```python
from build123d import *

# Parameters (mm, degrees)
SKETCH1_R           = 7.239
SKETCH1_W           = 3.175
SKETCH1_H           = 3.175
BOSS_EXTRUDE1_DEPTH = 6.35
SKETCH2_R           = 7.239
SKETCH2_W           = 3.175
SKETCH2_H           = 3.175
BOSS_EXTRUDE2_DEPTH = 0.254
SKETCH3_R           = 7.239
BOSS_EXTRUDE3_DEPTH = 6.35


with BuildPart() as part:
    # Sketch1 → Boss-Extrude1 (new body)
    with BuildSketch(Plane(origin=(0, 0, 0), x_dir=(1, 0, 0), z_dir=(0, 1, 0))):
        Circle(SKETCH1_R)
        Rectangle(SKETCH1_W, SKETCH1_H, mode=Mode.SUBTRACT)
    extrude(amount=BOSS_EXTRUDE1_DEPTH)

    # Sketch2 → Boss-Extrude2 (add)
    with BuildSketch(Plane(origin=(0, 6.35, 0), x_dir=(1, 0, 0), z_dir=(0, 1, 0))):
        Circle(SKETCH2_R)
        Rectangle(SKETCH2_W, SKETCH2_H, mode=Mode.SUBTRACT)
        Rectangle(SKETCH2_W, SKETCH2_H)
    extrude(amount=BOSS_EXTRUDE2_DEPTH)

    # Sketch3 → Boss-Extrude3 (add)
    with BuildSketch(Plane(origin=(0, 6.604, 0), x_dir=(1, 0, 0), z_dir=(0, 1, 0))):
        Circle(SKETCH3_R)
        Polygon((-1, -1), (-3, -1), (-3, 1), (-1, 1), (-1, 3), (1, 3), (1, 1), (3, 1), (3, -1), (1, -1), (1, -3), (-1, -3), align=None, mode=Mode.SUBTRACT)
    extrude(amount=BOSS_EXTRUDE3_DEPTH)


solid = part.part
```
Work out the finished part from the listing and answer in its coordinate system (mm). A direction names the side the tool comes from. Coordinates: 2 decimals unless noted, no trailing zeros. Order: outer loops, then holes, each group sorted by start corner. A loop starts at its lowest first (then second) coordinate and runs counter-clockwise, first axis right, second up. Notation, with made-up numbers: M -32,-35.5 L 10,-35.5 A28 cw 10,-11.5 Z; hole C -11,-26.5 d2. An arc over 180 degrees is marked long. Use CSV: the item, a comma, the result in double quotes.
1) For faces 4 (the face through (1.588, 3, 0)), 5 (the face through (-2, 0, 0)), 6 (the face through (-2, 10, -1)), determine the directions among +Z, -Z, +X, -X, +Y, -Y from which every point of the face is accessible in a straight line to the end or side of a thin tool.
Worked out:
face 4,"-Y"
face 5,"+Z, -Z, +X, -X, -Y"
face 6,"+Y"
2) Consider line 1 (X direction, y = 10, z = 0.25); line 2 (X direction, y = 7, z = 1.75); line 3 (Y direction, x = 2.75, z = -0.5). Determine where each line is inside the solid, lowest interval first. Write a range as [from, to].
Worked out:
line 1,"x = [-7.23, -3], [3, 7.23]"
line 2,"x = [-7.02, -1], [1, 7.02]"
line 3,"y = [0, 6.6]"
3) Determine the mould class of faces 1 (the face through (-3, 10, 0)), 2 (the face through (2, 12.954, 2)), 3 (the face through (-0.942, 6.386, -7.177)) for opening direction Z: released by +Z, released by -Z, zero draft, split by the parting line, or undercut.
Worked out:
face 1,"undercut"
face 2,"zero draft"
face 3,"split by the parting line"
4) Section B-B on y = 12.25 is taken. Write down the section's boundary in (x, z).
Worked out:
outline,"C 0,0 d14.48; hole M -3,-1 L -1,-1 L -1,-3 L 1,-3 L 1,-1 L 3,-1 L 3,1 L 1,1 L 1,3 L -1,3 L -1,1 L -3,1 Z"
5) Section A-A on z = 0 is taken. Write down the section's boundary in (x, y).
Worked out:
outline,"M -7.24,0 L -1.59,0 L -1.59,6.35 L 1.59,6.35 L 1.59,0 L 7.24,0 L 7.24,12.95 L 3,12.95 L 3,6.6 L -3,6.6 L -3,12.95 L -7.24,12.95 Z"
6) Flat-ended cylindrical pins translate along their axes: pin 1 Ø1.6 at (x, y) = (-2.5, 9) entering from -Z; pin 2 Ø1 at (x, z) = (0, 0.5) entering from -Y; pin 3 Ø0.6 at (y, z) = (8.5, -0.5) entering from +X. Find the tip coordinate at first contact, or state that the pin passes through.
Worked out:
pin 1,"stops at z = -7.04"
pin 2,"stops at y = 6.35"
pin 3,"stops at x = 7.24"
7) Section D-D on y = 2 is taken. Write down the section's boundary in (x, z).
Worked out:
outline,"C 0,0 d14.48; hole M -1.59,-1.59 L 1.59,-1.59 L 1.59,1.59 L -1.59,1.59 Z"
8) Section C-C on x = 0 is taken. Write down the section's boundary in (y, z), plus the area to 3 significant figures.
Worked out:
outline,"M 0,-7.24 L 12.95,-7.24 L 12.95,-3 L 6.6,-3 L 6.6,3 L 12.95,3 L 12.95,7.24 L 0,7.24 L 0,1.59 L 6.35,1.59 L 6.35,-1.59 L 0,-1.59 Z"
area,"129 mm^2"
